Input: part model. Units: mm. Frame: model coordinates. Give positions to 0.01 mm unless a question says otherwise; leave off trailing zeros. Order: outer loops, then holes, each group sorted by start corner. A loop starts at its lowest first (then second) coordinate and runs counter-clockwise, first axis right, second up. Notation, with made-up numbers: M 20,74.25 L 31,74.25 A21 ccw 31,82.25 Z; hole C 6,49 d9. An arc over 180 degrees is marked long. Use a Markdown table: item, result.
from build123d import *

# Parameters (mm, degrees)
F0_W = 40
F0_H = 40


with BuildPart() as f2:
    # F2: sweep along a path in F1
    with BuildLine(Plane.XZ) as f2_path:
        Line((0, 0), (0, 2240))
        Line((0, 2240), (1500, 2240))
        Line((1500, 2240), (1500, 0))
    # F0 (on Top) → F2 (sweep)
    with BuildSketch(Plane.XY):
        Rectangle(F0_W, F0_H)
    sweep(path=f2_path.line, transition=Transition.RIGHT)


solid = f2.part
1) Cut plane B-B on y = -7.5. Return loops of the section in (x, z), and give its area (3 significant figures).
Response values:
| item | result |
|---|---|
| outline | M -20,0 L 20,0 L 20,2220 L 1480,2220 L 1480,0 L 1520,0 L 1520,2260 L -20,2260 Z |
| area | 239,000 mm² |
2) Cut plane C-C on x = 717. Return loops of the section in (y, z).
Response values:
| item | result |
|---|---|
| outline | M -20,2220 L 20,2220 L 20,2260 L -20,2260 Z |
3) Cut plane A-A on z = 894.5. Return loops of the section in (x, y).
Response values:
| item | result |
|---|---|
| outline | M -20,-20 L 20,-20 L 20,20 L -20,20 Z; M 1480,-20 L 1520,-20 L 1520,20 L 1480,20 Z |
4) Material intervals for line 1 (X direction, y = 12, z = 513); line 2 (Z direction, x = 194.5, y = -1), sorted ascending. Write a range as from..to.
Response values:
| item | result |
|---|---|
| line 1 | x = -20..20, 1480..1520 |
| line 2 | z = 2220..2260 |
